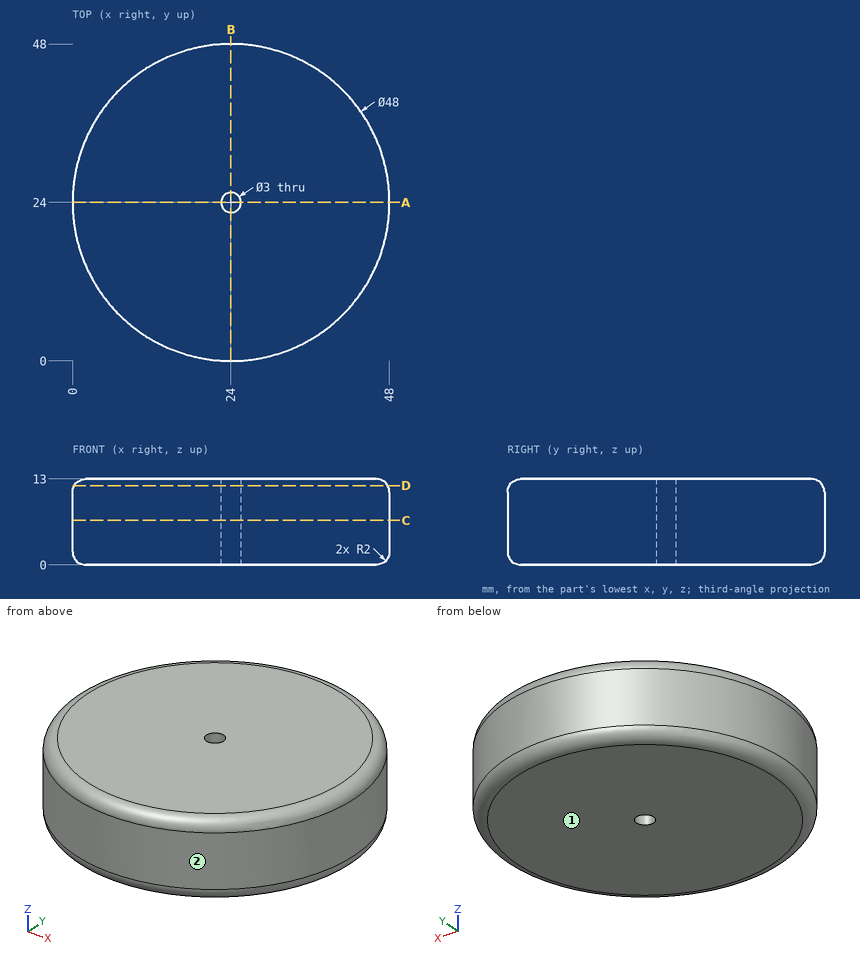
Part print with two shaded views. Sizes in mm from the minimum x, y, z corner. Round coordinates to 2 decimals unless told otherwise and drop trailing zeros. Order: outer loops, then holes, each group sorted by start corner. A loop starts at its lowest first (then second) coordinate and runs counter-clockwise, first axis right, second up. Notation, with made-up numbers: M 35.25,79.25 L 56.25,79.25 A26 cw 56.25,117.25 Z; hole C -36,55.25 d4. An arc over 180 degrees is marked long. Answer in a Markdown table with one row per item. Add a question column.
Q1. Wall check: L1, parallel to Y at x = 24, z = 4; L2, parallel to Y at x = 5, z = 7.75; L3, parallel to Y at x = 42.5, z = 11.75. Give the ranges that are in metal, low to high. Write a range as from..to.
Q2. Cut at D-D on z = 12. Give the cut face in (x, y), and give its area (3 significant figures).
Q3. Cut at A-A on y = 24. Give the cut face in (x, z), and give its area (3 significant figures).
Q4. Pin check, flat tips, straight feed: pin 1 (2 mm diameter, centred on x = 7, z = 5.5, fed in from +Y); pin 2 (5 mm diameter, centred on x = 28.5, z = 11.5, fed in from -Y); pin 3 (4 mm diameter, centred on y = 32.5, z = 10, fed in from -X). Stop position of each tip, or through.
Q5. Mould opens along X. For the marked faces 1 and 2 say: +X half, -X half, draft (parallel to the pull), parting line (faces both ways), or undercut.
Q6. Cut at C-C on z = 6.75. Give the cut face in (x, y).
Established:
| question | item | result |
|---|---|---|
| 1 | L1 | y = 0..22.5, 25.5..48 |
| 1 | L2 | y = 9.34..38.66 |
| 1 | L3 | y = 8.94..39.06 |
| 2 | outline | C 24,24 d47.46; hole C 24,24 d3 |
| 2 | area | 1,760 mm2 |
| 3 | outline | M 0,2 A2 ccw 2,0 L 22.5,0 L 22.5,13 L 2,13 A2 ccw 0,11 Z; M 25.5,0 L 46,0 A2 ccw 48,2 L 48,11 A2 ccw 46,13 L 25.5,13 Z |
| 3 | area | 582 mm2 |
| 4 | pin 1 | stops at y = 41.89 |
| 4 | pin 2 | stops at y = 0.09 |
| 4 | pin 3 | stops at x = 0.9 |
| 5 | face 1 | draft |
| 5 | face 2 | parting line |
| 6 | outline | C 24,24 d48; hole C 24,24 d3 |
